```python
from build123d import *

# Parameters (mm, degrees)
BOSS_EXTRUDE1_DEPTH = 12.5
BOSS_EXTRUDE2_DEPTH = 4.3
SKETCH4_R           = 2.4
BOSS_EXTRUDE3_DEPTH = 3.5
CUT_EXTRUDE1_REACH  = 37.89


with BuildPart() as part:
    # Sketch1 → Boss-Extrude1 (new body)
    with BuildSketch(Plane.XY):
        Polygon((0, 0), (23.2, 0), (23.2, 16.4), (27.9, 16.4), (27.9, 18.8), (23.2, 18.8), (23.2, 23), (0, 23), (0, 18.8), (-4.7, 18.8), (-4.7, 16.4), (0, 16.4), align=None)
    extrude(amount=BOSS_EXTRUDE1_DEPTH)

    # Sketch3 → Boss-Extrude2 (add)
    with BuildSketch(Plane(origin=(0, 23, 0), x_dir=(1, 0, 0), z_dir=(0, 1, 0))):
        with BuildLine():
            Line((11.978219619, -8.75), (12.978219619, -8.75))
            ThreePointArc((12.978219619, -8.75), (15.478219619, -6.25), (12.978219619, -3.75))
            Line((12.978219619, -3.75), (11.978219619, -3.75))
            ThreePointArc((11.978219619, -3.75), (0, -6.25), (11.978219619, -8.75))
        make_face()
    extrude(amount=BOSS_EXTRUDE2_DEPTH)

    # Sketch4 → Boss-Extrude3 (add)
    with BuildSketch(Plane(origin=(0, 27.3, 0), x_dir=(1, 0, 0), z_dir=(0, 1, 0))):
        with Locations(Location((6.25, -6.25, 0), (0, 0, 270))):
            Circle(SKETCH4_R)
    extrude(amount=BOSS_EXTRUDE3_DEPTH)

    # Sketch2 → Cut-Extrude1 (cut, up to next)
    with BuildSketch(Plane(origin=(0, 18.8, 0), x_dir=(1, 0, 0), z_dir=(0, 1, 0)), mode=Mode.PRIVATE) as cut_extrude1_sk1:
        with BuildLine():
            Line((27.9, -6.75), (27.9, -5.75))
            Line((27.9, -5.75), (26.9, -5.75))
            ThreePointArc((26.9, -5.75), (25.033974596, -6.25), (26.9, -6.75))
            Line((26.9, -6.75), (27.9, -6.75))
        make_face()
    cut_extrude1_tool1 = extrude(cut_extrude1_sk1.sketch, amount=-CUT_EXTRUDE1_REACH, mode=Mode.PRIVATE) & part.part
    # Sketch2 → Cut-Extrude1 (cut, up to next)
    with BuildSketch(Plane(origin=(0, 18.8, 0), x_dir=(1, 0, 0), z_dir=(0, 1, 0)), mode=Mode.PRIVATE) as cut_extrude1_sk2:
        with BuildLine():
            Line((-4.7, -6.75), (-3.7, -6.75))
            ThreePointArc((-3.7, -6.75), (-1.833974596, -6.25), (-3.7, -5.75))
            Line((-3.7, -5.75), (-4.7, -5.75))
            Line((-4.7, -5.75), (-4.7, -6.75))
        make_face()
    cut_extrude1_tool2 = extrude(cut_extrude1_sk2.sketch, amount=-CUT_EXTRUDE1_REACH, mode=Mode.PRIVATE) & part.part
    add(cut_extrude1_tool1.solids().sort_by_distance((26.35061, 18.8, 6.25))[0], mode=Mode.SUBTRACT)
    add(cut_extrude1_tool2.solids().sort_by_distance((-3.15061, 18.8, 6.25))[0], mode=Mode.SUBTRACT)


solid = part.part
```
Geometry: final body of the model. Coordinates: model frame, mm. A direction names the side the tool comes from. Round coordinates to 2 decimals unless told otherwise and drop trailing zeros. Write each loop counter-clockwise with the first axis right and the second up, starting at its lowest first coordinate (ties: lowest second). Pieces come first, ordered by that corner, then holes.
Item 1: Material intervals for L1, parallel to X at y = 18, z = 7; L2, parallel to X at y = 17.95, z = 6.25; L3, parallel to Y at x = 12, z = 3, sorted ascending.
Item 2: Section query B-B (z = 10.25). Return loops of the section in (x, y), plus the area to 3 significant figures.
Item 3: Mould query, pull axis X, two halves, no side actions, for faces 1 (the face through (25.035, 17.617, 6.213)), 2 (the face through (-4.7, 18, 10)), 3 (the face through (12.5, 25.1, 3.75)), 4 (the face through (7.87, 29.03, 4.48)). Classes: +X half, -X half, draft (parallel to the pull), parting line (faces both ways), or undercut.
Item 4: Section query D-D (z = 1.75). Return loops of the section in (x, y).
Item 5: Set-up query: faces 5 (the face through (9, 27.3, 6)), 6 (the face through (24, 16.4, 6)), 7 (the face through (27.4, 17.6, 5.75)), 8 (the face through (12.5, 25.1, 8.75)). Return all of +Z, -Z, +X, -X, +Y, -Y with unobstructed straight access to the full face (end or side cutting, diameter ignored); none if empty.
Item 6: Section query A-A (y = 18). Return loops of the section in (x, z), plus the area to 3 significant figures.
Item 7: Pin query (flat end, axial travel): P1, Ø1.5, axis at x = -0.5, y = 23, coming from the +Z side; P2, Ø1.6, axis at x = -2.83, z = 6.25, coming from the -Y side; P3, Ø2, axis at y = 20, z = 8.5, coming from the +X side; P4, Ø1.5, axis at x = 1.5, z = 7, coming from the +Y side. Return the tip coordinate at first contact, or that it passes through.
Item 8: Section query C-C (y = 28). Return loops of the section in (x, z), plus the area to 3 significant figures.
Completed:
1. L1: x = -4.7 to -3.5, -2.17 to 25.37, 26.7 to 27.9
1. L2: x = -1.83 to 25.03
1. L3: y = 0 to 23
2. outline: (-4.7, 16.4) - (0, 16.4) - (0, 0) - (23.2, 0) - (23.2, 16.4) - (27.9, 16.4) - (27.9, 18.8) - (23.2, 18.8) - (23.2, 23) - (11.05, 23) - (11.05, 27.3) - (1.45, 27.3) - (1.45, 23) - (0, 23) - (0, 18.8) - (-4.7, 18.8) - close
2. area: 597 mm2
3. face 1: undercut
3. face 2: -X half
3. face 3: draft
3. face 4: parting line
4. outline: (-4.7, 16.4) - (0, 16.4) - (0, 0) - (23.2, 0) - (23.2, 16.4) - (27.9, 16.4) - (27.9, 18.8) - (23.2, 18.8) - (23.2, 23) - (10.59, 23) - (10.59, 27.3) - (1.91, 27.3) - (1.91, 23) - (0, 23) - (0, 18.8) - (-4.7, 18.8) - close
5. face 5: +Y
5. face 6: +Z, -Z, +X, -Y
5. face 7: +X, +Y, -Y
5. face 8: +Z, +X, +Y
6. outline: (-4.7, 0) - (27.9, 0) - (27.9, 5.75) - (26.9, 5.75) arc R1 cw (long way) to (26.9, 6.75) - (27.9, 6.75) - (27.9, 12.5) - (-4.7, 12.5) - (-4.7, 6.75) - (-3.7, 6.75) arc R1 cw (long way) to (-3.7, 5.75) - (-4.7, 5.75) - close
6. area: 399 mm2
7. P1: stops at z = 12.5
7. P2: passes through
7. P3: stops at x = 23.2
7. P4: stops at y = 27.3
8. outline: circle Ø4.8 at (6.25, 6.25)
8. area: 18.1 mm2
